Input: dimensioned drawing with shaded views. Units: mm. Origin: part minimum x, y, z. A direction names the side the tool comes from. Give positions to 0.01 mm unless a question says otherwise; leave off trailing zeros. Write each loop counter-clockwise with the first axis right and the second up, starting at its lowest first coordinate (ties: lowest second). Pieces come first, ordered by that corner, then holes. Notation, with made-up numbers: (29.25, 51) -> (76.25, 51) arc R23 ccw to (76.25, 85) -> close; hole circle Ø11 at (47, 87.25). An arc over 180 degrees is marked (long way). Return JSON: item names as keys, results as strings. Group by question number.
Item 1: Pin query (flat end, axial travel): P1, Ø12.5, axis at x = 42, y = 34, coming from the +Z side; P2, Ø2, axis at y = 49, z = 59.5, coming from the +X side; P3, Ø9, axis at x = 78.5, y = 40, coming from the +Z side; P4, Ø24, axis at x = 120, z = 40, coming from the -Y side. Return the tip coordinate at first contact, or that it passes through.
Item 2: Section B-B, the plane y = 9.5. Return loops of the section in (x, z), then the cut area to 3 significant figures.
Item 3: Section A-A, the plane x = 120. Return loops of the section in (y, z).
Item 4: Line query: line 1 (Z direction, x = 120, y = 20); line 2 (Z direction, x = 69, y = 40); line 3 (Z direction, x = 52, y = 48). Output: solid intervals per line, ascending. Write a range as [from, to].
Item 5: Section C-C, the plane z = 33.5. Return loops of the section in (x, y).
Item 6: Set-up query: the marked faces 5, 6 and 7. Return all of +Z, -Z, +X, -X, +Y, -Y with unobstructed straight access to the full face (end or side cutting, diameter ignored); none if empty.
Item 7: Mould query, pull axis X, two halves, no side actions, for the marked faces 1, 2, 3 and 4. Classes: released by +X, released by -X, zero draft, split by the parting line, or undercut.
Item 8: Section D-D, the plane x = 96.5. Return loops of the section in (y, z).
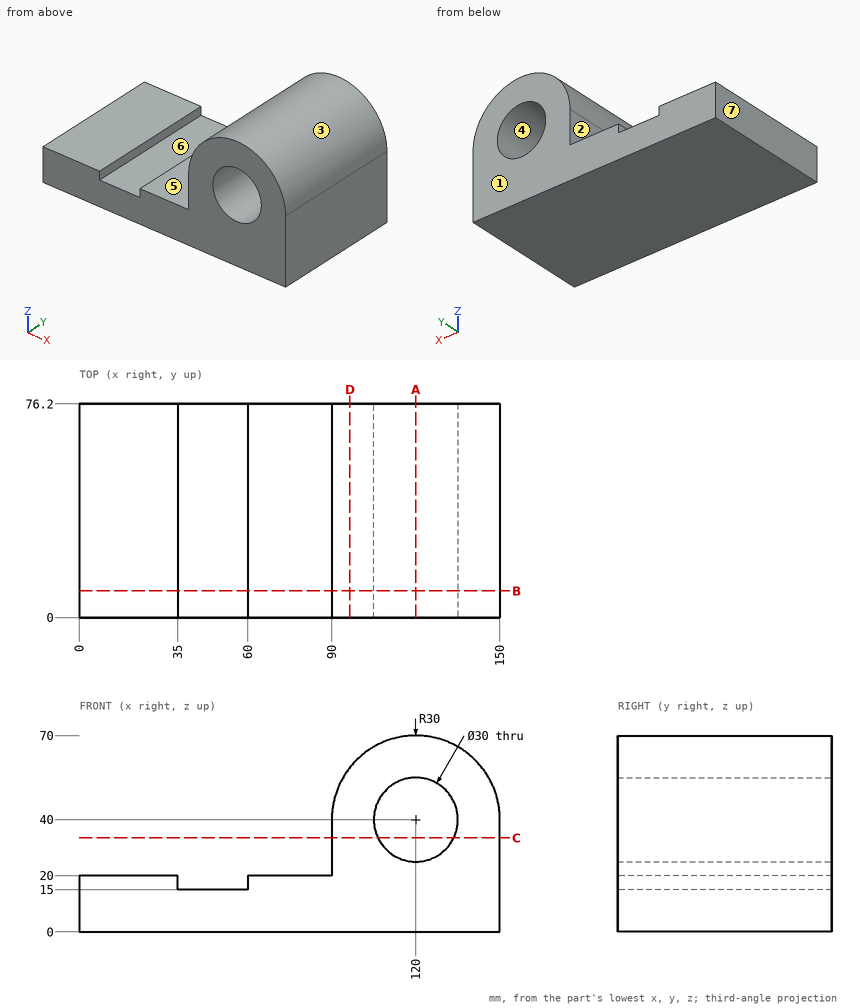
Answer below:
{
 "1": {"P1": "stops at z = 15", "P2": "stops at x = 143.62", "P3": "stops at z = 20", "P4": "passes through"},
 "2": {"outline": "(0, 0) -> (150, 0) -> (150, 40) arc R30 ccw to (90, 40) -> (90, 20) -> (60, 20) -> (60, 15) -> (35, 15) -> (35, 20) -> (0, 20) -> close; hole circle Ø30 at (120, 40)", "area": "4,780 mm2"},
 "3": {"outline": "(0, 0) -> (76.2, 0) -> (76.2, 25) -> (0, 25) -> close; (0, 55) -> (76.2, 55) -> (76.2, 70) -> (0, 70) -> close"},
 "4": {"line 1": "z = [0, 25], [55, 70]", "line 2": "z = [0, 20]", "line 3": "z = [0, 15]"},
 "5": {"outline": "(90, 0) -> (106.48, 0) -> (106.48, 76.2) -> (90, 76.2) -> close; (133.52, 0) -> (150, 0) -> (150, 76.2) -> (133.52, 76.2) -> close"},
 "6": {"face 5": "+Z, -X, +Y, -Y", "face 6": "+Z, +Y, -Y", "face 7": "+Z, -Z, -X, +Y, -Y"},
 "7": {"face 1": "zero draft", "face 2": "released by -X", "face 3": "split by the parting line", "face 4": "undercut"},
 "8": {"outline": "(0, 0) -> (76.2, 0) -> (76.2, 58.65) -> (0, 58.65) -> close"}
}
